CAD build for the part. Positions are in the model's coordinates, mm. Face numbers are marked on the shaded views. Round coordinates to 2 decimals unless told otherwise and drop trailing zeros. Order: outer loops, then holes, each group sorted by start corner. A loop starts at its lowest first (then second) coordinate and runs counter-clockwise, first axis right, second up. Notation, with made-up numbers: (-32, 11.25) - (-18, 11.25) arc R30 cw to (-18, 35.25) - close; hole circle Ø1 at (-24, -26.5). An arc over 180 degrees is marked (long way). Write item = value, one per line.
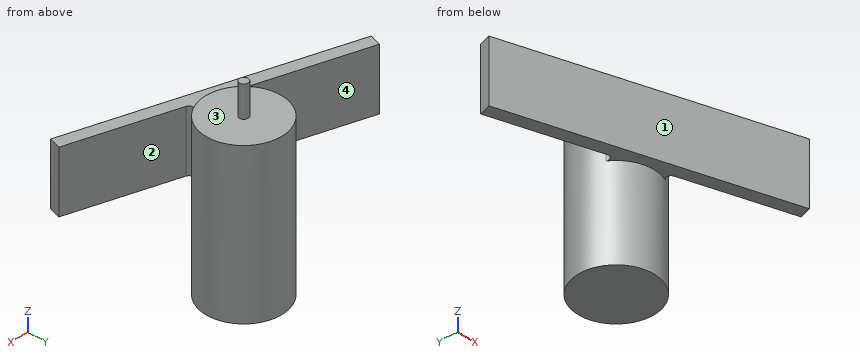
from build123d import *

# Parameters (mm, degrees)
SKETCH1_R                = 22
BOSS_EXTRUDE1_DEPTH      = 91
SKETCH2_R                = 2.525052574
BOSS_EXTRUDE2_DEPTH      = 18
SKETCH4_W                = 155
SKETCH4_H                = 35.569912337
BOSS_EXTRUDE3_DEPTH      = 6
BOSS_EXTRUDE3_DEPTH_BACK = 1
FILLET1_R                = 2.5
FILLET2_R                = 2.5


with BuildPart() as part:
    # Sketch1 → Boss-Extrude1 (new body)
    with BuildSketch(Plane.XY):
        with Locations((-5.492733953, -4.838837054)):
            Circle(SKETCH1_R)
    extrude(amount=BOSS_EXTRUDE1_DEPTH)

    # Sketch2 → Boss-Extrude2 (add)
    with BuildSketch(Plane.XY.offset(91)):
        with Locations((-5.492733953, -4.838837054)):
            Circle(SKETCH2_R)
    extrude(amount=BOSS_EXTRUDE2_DEPTH)

    # Sketch4 → Boss-Extrude3 (add, two sides)
    with BuildSketch(Plane(origin=(-12.142972716, -25.809633996, 91), x_dir=(-0.953218043, 0.30228358, 0), z_dir=(-0.30228358, -0.953218043, 0))) as boss_extrude3_sk:
        with Locations((0, 19.988267876)):
            Rectangle(SKETCH4_W, SKETCH4_H)
    extrude(amount=BOSS_EXTRUDE3_DEPTH)
    extrude(boss_extrude3_sk.sketch, amount=-BOSS_EXTRUDE3_DEPTH_BACK)

    # Fillet1
    fillet1_edges = [part.edges().sort_by_distance(p)[0] for p in [
        (-5.59002042, -26.838621947, 71.011732124),
    ]]
    fillet(fillet1_edges, radius=FILLET1_R)

    # Fillet2
    fillet2_edges = [part.edges().sort_by_distance(p)[0] for p in [
        (-18.091357852, -22.87420996, 71.011732124),
    ]]
    fillet(fillet2_edges, radius=FILLET2_R)


solid = part.part
(1) Pull direction X, two halves, no side cores. Call the marked faces 1, 2, 3 and 4: released by +X, released by -X, zero draft, split by the parting line, or undercut.
Solved:
face_1 = released by -X
face_2 = released by +X
face_3 = zero draft
face_4 = undercut
(2) Drop a flat-ended pin along its axis: pin 1 (6 mm diameter, centred on y = -3, z = 15, fed in from +X). Give the stop position or say it passes through.
Solved:
pin_1 = 16.51
(3) Probe line 1 along Z through (x, y) = (14.5, 2); line 2 along X through (y, z) = (13.5, 63); line 3 along X through (y, z) = (8, 23.5). List the from-to ranges inside material, lowest first.
Solved:
line_1 = 0 to 91
line_2 = -17.65 to 6.66
line_3 = -23.36 to 12.37
(4) Band-saw the part on B-B on z = 59. List the corners of the cut face in (x, y), plus the area to 3 significant figures.
Solved:
outline = (-87.83, -8.1) - (59.92, -54.96) - (62.03, -48.28) - (3.47, -29.71) arc R2.5 cw to (3.23, -25.03) arc R22 ccw (long way) to (-24.26, -16.31) arc R2.5 cw to (-27.15, -20) - (-85.72, -1.43) - close
area = 2,620 mm²
(5) Band-saw the part on D-D on y = 3. List the corners of the cut face in (x, z), plus the area to 3 significant figures.
Solved:
outline = (-26.05, 0) - (15.06, 0) - (15.06, 91) - (-26.05, 91) - close
area = 3,740 mm²
(6) Band-saw the part on C-C on x = 48. List the corners of the cut face in (y, z).
Solved:
outline = (-51.18, 53.23) - (-43.83, 53.23) - (-43.83, 88.8) - (-51.18, 88.8) - close
(7) Band-saw the part on A-A on y = -11.5. List the corners of the cut face in (x, z), plus the area to 3 significant figures.
Solved:
outline = (-77.12, 53.23) - (-53.96, 53.23) - (-53.96, 88.8) - (-77.12, 88.8) - close; (-26.46, 0) - (15.47, 0) - (15.47, 91) - (-26.46, 91) - close
area = 4,640 mm²
